Print and shaded views of the part. All mm, measured from the part's lowest x, y and z. Coordinates: 2 decimals unless noted, no trailing zeros. Order: outer loops, then holes, each group sorted by start corner. A loop starts at its lowest first (then second) coordinate and runs counter-clockwise, first axis right, second up. Notation, with made-up numbers: (21.25, 6) -> (56.25, 6) arc R11 ccw to (56.25, 10) -> close; hole circle Ø1 at (27.5, 68.25). An arc over 180 degrees is marked (long way). Write item = value, one per line. Start each with the question number.
Q1. Mould opens along X. For the marked faces 1, 2, 3 and 4 say: +X half, -X half, draft (parallel to the pull), parting line (faces both ways), or undercut.
Q2. Flat gauge pins, fed straight in: pin 1 (1 mm diameter, centred on x = 7.5, y = 22, fed in from +Z); pin 2 (2 mm diameter, centred on x = 40.5, z = 1, fed in from +Y); pin 3 (9 mm diameter, centred on x = 25, y = 25, fed in from +Z); pin 4 (2 mm diameter, centred on x = 19.5, z = 4.5, fed in from +Y). Where does each tip first touch, or does it go through?
Q3. Cut at A-A, the plane y = 27. List the corners of the cut face in (x, z).
Q4. Wall check: line 1 (Y direction, x = 25, z = 2.25); line 2 (Y direction, x = 25, z = 5.3); line 3 (X direction, y = 21.5, z = 0.35). Give the ranges that are in metal, low to high. Write a range as from..to.
Q5. Cut at B-B, the plane x = 25. List the corners of the cut face in (y, z), plus the area to 3 significant figures.
Q6. Cut at D-D, the plane y = 44. List the corners of the cut face in (x, z).
Q7. Cut at C-C, the plane z = 5. List the corners of the cut face in (x, y).
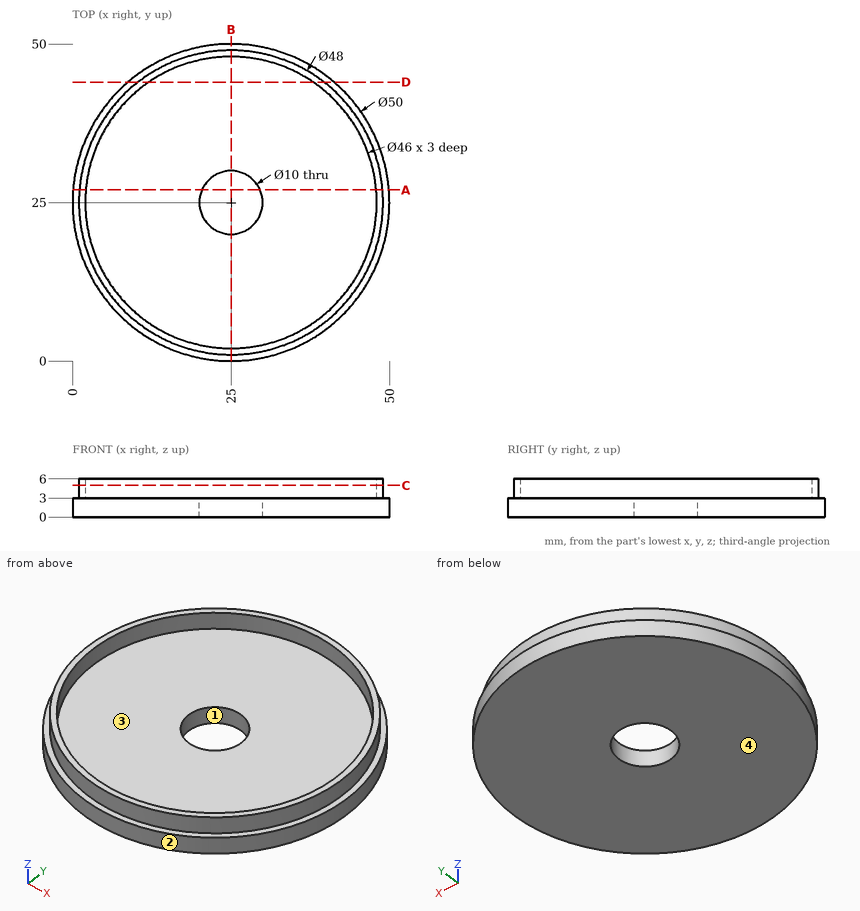
Here are the results:
q1.face_1 = undercut
q1.face_2 = parting line
q1.face_3 = undercut
q1.face_4 = draft
q2.pin_1 = 3
q2.pin_2 = 45.37
q2.pin_3 = through
q2.pin_4 = 48.57
q3.outline = (0.08, 0) -> (20.42, 0) -> (20.42, 3) -> (2.09, 3) -> (2.09, 6) -> (1.08, 6) -> (1.08, 3) -> (0.08, 3) -> close; (29.58, 0) -> (49.92, 0) -> (49.92, 3) -> (48.92, 3) -> (48.92, 6) -> (47.91, 6) -> (47.91, 3) -> (29.58, 3) -> close
q4.line_1 = 0..20, 30..50
q4.line_2 = 1..2, 48..49
q4.line_3 = 0.25..21.43, 28.57..49.75
q5.outline = (0, 0) -> (20, 0) -> (20, 3) -> (2, 3) -> (2, 6) -> (1, 6) -> (1, 3) -> (0, 3) -> close; (30, 0) -> (50, 0) -> (50, 3) -> (49, 3) -> (49, 6) -> (48, 6) -> (48, 3) -> (30, 3) -> close
q5.area = 126 mm²
q6.outline = (8.75, 0) -> (41.25, 0) -> (41.25, 3) -> (39.66, 3) -> (39.66, 6) -> (37.96, 6) -> (37.96, 3) -> (12.04, 3) -> (12.04, 6) -> (10.34, 6) -> (10.34, 3) -> (8.75, 3) -> close
q7.outline = circle Ø48 at (25, 25); hole circle Ø46 at (25, 25)
